Can you work these out from the drawing? Everything is in mm from the part's minimum corner. Coordinates: 2 decimals unless noted, no trailing zeros. Order: outer loops, then holes, each group sorted by start corner. A loop starts at its lowest first (then second) coordinate and runs counter-clockwise, first axis right, second up. Notation, with made-up numbers: (-11.5, 52.25) - (13.5, 52.25) arc R30 ccw to (13.5, 89.25) - close; hole circle Ø5 at (51, 8). An arc over 180 degrees is marked (long way). Use a Markdown table: item, result. Add a question column.
(1) I want a section at A-A (z = 90). List the corners of the cut face in (x, y) for me.
(2) I want a section at C-C (y = 0.75). List the corners of the cut face in (x, z) for me.
(3) I want a section at B-B (x = 7). List the corners of the cut face in (y, z) for me, and give its area (3 significant figures).
(4) I want a section at D-D (x = 12). List the corners of the cut face in (y, z) for me, and give its area (3 significant figures).
(5) If I drill on L1, parallel to Z at x = 7, y = 1.85; L2, parallel to X at y = 3.1, z = 90; L3, parallel to X at y = 0.95, z = 14.5, over which ranges is the centre line in solid material (lowest first)? Write a range as [from, to].
(6) For pin 1 Ø1.5 at (x, y) = (12.5, 1.5) entering from -Z, with a flat end and sliding along its axis, tell me the tip position at first contact or that it passes through.
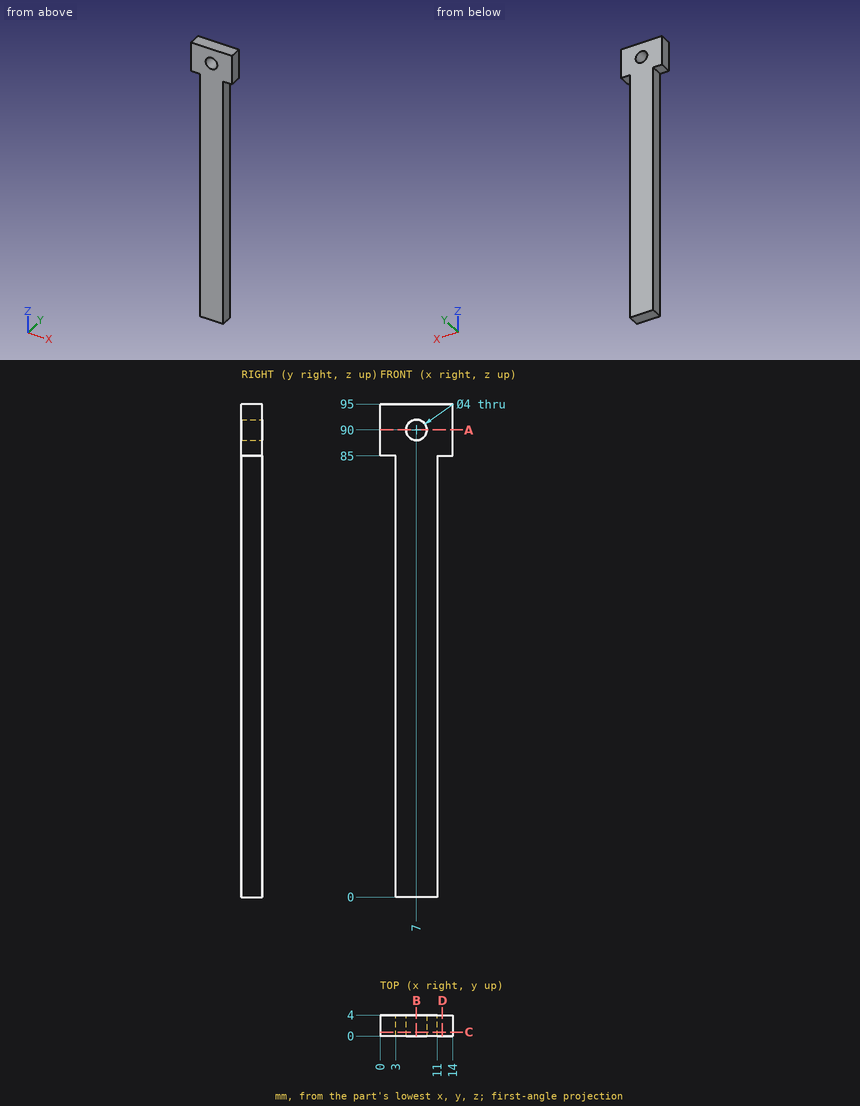
Answers follow:
| question | item | result |
|---|---|---|
| 1 | outline | (0, 0) - (5, 0) - (5, 4) - (0, 4) - close; (9, 0) - (14, 0) - (14, 4) - (9, 4) - close |
| 2 | outline | (0, 85) - (3, 85) - (3, 0) - (11, 0) - (11, 85) - (14, 85) - (14, 95) - (0, 95) - close; hole circle Ø4 at (7, 90) |
| 3 | outline | (0, 0) - (4, 0) - (4, 88) - (0, 88) - close; (0, 92) - (4, 92) - (4, 95) - (0, 95) - close |
| 3 | area | 364 mm² |
| 4 | outline | (0, 85) - (4, 85) - (4, 95) - (0, 95) - close |
| 4 | area | 40.0 mm² |
| 5 | L1 | z = [0, 88], [92, 95] |
| 5 | L2 | x = [0, 5], [9, 14] |
| 5 | L3 | x = [3, 11] |
| 6 | pin 1 | stops at z = 85 |
